Design review of the part built by this model. Coordinates are the model's own, in mm. Coordinates: 2 decimals unless noted, no trailing zeros. Order: outer loops, then holes, each group sorted by start corner. A loop starts at its lowest first (then second) coordinate and runs counter-clockwise, first axis right, second up. Notation, with made-up numbers: (51.5, 42) -> (91.5, 42) arc R23 ccw to (91.5, 80) -> close; hole circle Ø4 at (9.25, 33.5). An arc over 180 degrees is marked (long way). Use a Markdown table: item, result. Add a question column.
Q1. Add section C-C (x = 5.5). State the section outline as (y, z) points.
Q2. The part is to be moulded in two halves that separate along Z. For faces 1 (the face through (-10.189, 88.03, 45.882)), 2 (the face through (-34, 0, 33)), 3 (the face through (46.06, 160.2, -11.38)), 4 (the face through (-10.84, 89.85, 48.81)), say which applies: pulls with the +Z half, pulls with the -Z half, needs draft (parallel to the pull), parting line crosses it, or undercut.
Q3. Add section B-B (y = 77). State the section outline as (x, z) points.
Q4. Wall thickness on probe 1 along X at (y, z) = (142, 0); probe 2 along Z at (x, y) = (-5, 22): over which ranges is each line inside the solid? List them lowest first.
Q5. Insertion check: pin 1 (5 mm diameter, centred on x = 35.5, y = 42.5, fed in from +Z); pin 2 (4 mm diameter, centred on x = 4.5, y = 136, fed in from +Z); pin 3 (12 mm diameter, centred on x = -3.5, y = 69.5, fed in from +Z). Each pin has a flat end and moves straight along its axis. Give the tip position at first contact, or say it passes through.
Q6. Add section A-A (x = 25.5). State the section outline as (y, z) points, then the cut area to 3 significant figures.
from build123d import *

# Parameters (mm, degrees)
EXTRUDE_1_OUTLINE_R      = 50
EXTRUDE_1_OUTLINE_R_2    = 47
EXTRUDE_1_DEPTH          = 200
CUT_EXTRUDE_1_DEPTH      = 213.132034356
CUT_EXTRUDE_1_DEPTH_BACK = 213.132034356
SKETCH_2_R               = 62.5


# Read off the part's stored shape, not the designer's step: Вытянуть-Тонкостенный1
with BuildPart() as part:
    # Вытянуть-Тонкостенный1 outline → Вытянуть-Тонкостенный1 (new body)
    with BuildSketch(Plane(origin=(0, 0, 0), x_dir=(1, 0, 0), z_dir=(0, 1, 0))):
        Circle(EXTRUDE_1_OUTLINE_R)
        Circle(EXTRUDE_1_OUTLINE_R_2, mode=Mode.SUBTRACT)
    extrude(amount=EXTRUDE_1_DEPTH)

    # Эскиз2 → Вырез-Вытянуть1 (cut, two sides: drawn at the far end of the back side and taken through both)
    with BuildSketch(Plane(origin=(0, 0, 0), x_dir=(1, 0, 0), z_dir=(0, -0.5735764363510444, -0.819152044288993)).offset(-CUT_EXTRUDE_1_DEPTH_BACK)):
        with Locations((0, -180)):
            Circle(SKETCH_2_R)
    extrude(amount=CUT_EXTRUDE_1_DEPTH + CUT_EXTRUDE_1_DEPTH_BACK, mode=Mode.SUBTRACT)


solid = part.part
Established:
| question | item | result |
|---|---|---|
| 1 | outline | (0, -49.7) -> (108.94, -49.7) -> (111.05, -46.68) -> (0, -46.68) -> close; (0, 46.68) -> (176.42, 46.68) -> (178.53, 49.7) -> (0, 49.7) -> close |
| 2 | face 1 | undercut |
| 2 | face 2 | needs draft |
| 2 | face 3 | pulls with the -Z half |
| 2 | face 4 | parting line crosses it |
| 3 | outline | circle Ø100 at (0, 0); hole circle Ø94 at (0, 0) |
| 4 | probe 1 | -50 to -47, 47 to 50 |
| 4 | probe 2 | -49.75 to -46.73, 46.73 to 49.75 |
| 5 | pin 1 | z = 37.56 |
| 5 | pin 2 | z = 49.94 |
| 5 | pin 3 | z = 50 |
| 6 | outline | (0, -43.01) -> (119.97, -43.01) -> (122.44, -39.48) -> (0, -39.48) -> close; (0, 39.48) -> (177.73, 39.48) -> (180.2, 43.01) -> (0, 43.01) -> close |
| 6 | area | 1,060 mm^2 |
